Input: dimensioned drawing with shaded views. Units: mm. Origin: part minimum x, y, z. A direction names the side the tool comes from. Round coordinates to 2 decimals unless told otherwise and drop trailing zeros. Loops run counter-clockwise (first coordinate to the right, second up) from the corner with the lowest first, then second, coordinate; pieces in that order, holes last. Notation, with made-up numbers: (14.25, -19) - (30.25, -19) arc R11 ccw to (30.25, 1) - close; hole circle Ø11 at (63.25, -23). An arc over 180 degrees is marked (long way). Answer as CSV lines item,"result".
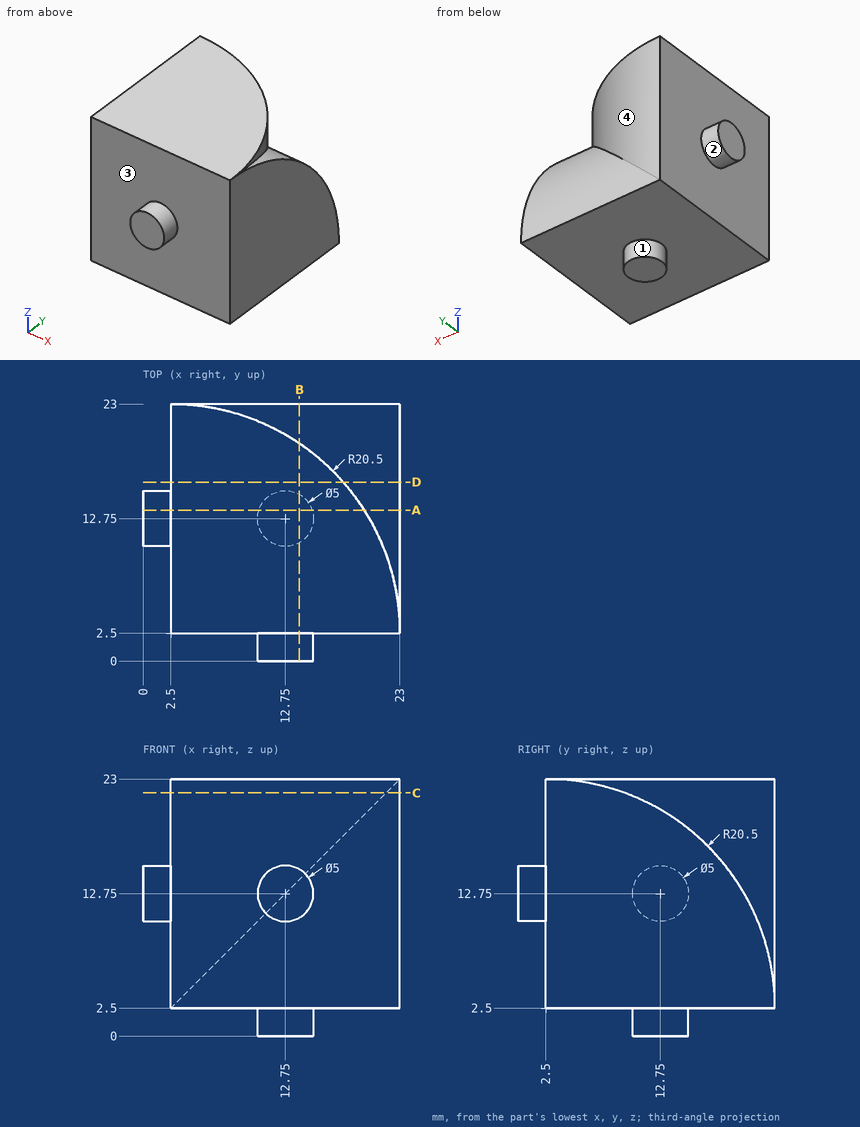
(1) Section C-C (z = 21.75). Output: boundary loops of the cut face in (x, y), and give its area (3 significant figures).
Findings below:
outline,"(2.5, 2.5) - (23, 2.5) - (23, 9.55) - (21.75, 9.55) arc R20.5 ccw to (2.5, 23) - close"
area,"333 mm2"
(2) Access query for the marked faces 1, 2, 3 and 4. Directions: +Z, -Z, +X, -X, +Y, -Y. A direction counts if a zero-diameter tool reaches every point of the face in a straight line with its end or side. Return the directions, or none.
Findings below:
face 1,"-Z"
face 2,"-X"
face 3,"-Y"
face 4,"+Z, +X, +Y"
(3) Section B-B (x = 14). Output: boundary loops of the cut face in (y, z).
Findings below:
outline,"(0, 10.58) - (2.5, 10.58) - (2.5, 2.5) - (10.58, 2.5) - (10.58, 0) - (14.92, 0) - (14.92, 2.5) - (23, 2.5) arc R20.5 ccw to (19.47, 14) - (19.47, 23) - (2.5, 23) - (2.5, 14.92) - (0, 14.92) - close"
(4) Section D-D (y = 16). Output: boundary loops of the cut face in (x, z), and give its area (3 significant figures).
Findings below:
outline,"(2.5, 2.5) - (23, 2.5) - (23, 17.93) - (17.93, 17.93) - (17.93, 23) - (2.5, 23) - close"
area,"395 mm2"
(5) Section A-A (y = 13.5). Output: boundary loops of the cut face in (x, z).
Findings below:
outline,"(0, 10.37) - (2.5, 10.37) - (2.5, 2.5) - (10.37, 2.5) - (10.37, 0) - (15.13, 0) - (15.13, 2.5) - (23, 2.5) - (23, 19.8) - (19.8, 19.8) - (19.8, 23) - (2.5, 23) - (2.5, 15.13) - (0, 15.13) - close"
(6) Material intervals for line 1 along Z through (x, y) = (3.5, 20.5); line 2 along Y through (x, z) = (7.25, 5.25), sorted ascending.
Findings below:
line 1,"2.5 to 23"
line 2,"2.5 to 22.81"
(7) Pin query (flat end, axial travel): P1, Ø2, axis at x = 19.5, z = 7, coming from the +Y side; P2, Ø2, axis at x = 7.5, z = 11, coming from the +Y side; P3, Ø10, axis at x = 8, y = 5, coming from the -Z side. Return the tip coordinate at first contact, or that it passes through.
Findings below:
P1,"y = 22.7"
P2,"y = 22.61"
P3,"z = 2.5"
